Design review of the part built by this model. Coordinates are the model's own, in mm. A direction names the side the tool comes from. Coordinates: 2 decimals unless noted, no trailing zeros. Loops run counter-clockwise (first coordinate to the right, second up) from the corner with the lowest first, then second, coordinate; pieces in that order, holes last. Notation, with made-up numbers: (19, 64) -> (75, 64) arc R4 ccw to (75, 69) -> close; hole circle Ø7 at (81, -4). An arc over 180 degrees is marked (long way). Use one line per item in the form item = value. Start each with the question number.
1. Machinability: for faces 1 (the face through (-6, -0.3, 3)), 2 (the face through (6, 2.2, 3)), 3 (the face through (-6.5, -2.2, 3)), which of the approach directions +Z, -Z, +X, -X, +Y, -Y give a long, thin tool a straight path to every point of the face, cutting with its end or side? Answer none if there is none.
2. Consider section B-B (y = 1). State the section outline as (x, z) points, then the cut area to 3 significant figures.
3. Wall thickness on line 1 (Y direction, x = -9.5, z = 1.25); line 2 (X direction, y = -1.75, z = 4.25); line 3 (Y direction, x = 0.25, z = 3): over which ranges is each line inside the solid? List them lowest first. Write a range as from..to.
4. Consider section A-A (x = 0). State the section outline as (y, z) points, then the cut area to 3 significant figures.
5. The part is to be moulded in two halves that separate along X. For faces 4 (the face through (3, 3, 0)), 5 (the face through (-7.384, -1.237, 1.735)), 6 (the face through (0, 5, 3)), say which applies: released by +X, released by -X, zero draft, split by the parting line, or undercut.
6. Consider section C-C (y = -3). State the section outline as (x, z) points.
7. Consider section D-D (x = -7.5). State the section outline as (y, z) points.
8. For pin 1 (1.8 mm diameter, centred on x = -7, z = 2, fed in from +Y); pin 2 (2.5 mm diameter, centred on x = 8.19, z = 3, fed in from -Y); pin 3 (3.5 mm diameter, centred on x = -8.19, z = 3, fed in from -Y); pin 4 (1.5 mm diameter, centred on y = 1.5, z = 2, fed in from -X), all flat-tipped, find the tip position at first contact; note any pin that passes through.
from build123d import *

# Parameters (mm, degrees)
EXTRUDE_1_DEPTH     = 6
CUT_EXTRUDE_1_DEPTH = 8.2
SKETCH_4_R          = 1.5
CUT_EXTRUDE_2_DEPTH = 8.2
FILLET_1_R          = 0.3


with BuildPart() as part:
    # 草图2 → 凸台-拉伸1 (new body)
    with BuildSketch(Plane.XY):
        with BuildLine():
            Line((-11.189988864, 0.3), (-11.189988864, 2.2))
            Line((-11.189988864, 2.2), (-4.489988864, 2.2))
            ThreePointArc((-4.489988864, 2.2), (0, 5), (4.489988864, 2.2))
            Line((4.489988864, 2.2), (11.189988864, 2.2))
            Line((11.189988864, 2.2), (11.189988864, 0))
            Line((11.189988864, 0), (4, 0))
            ThreePointArc((4, 0), (0.150105729, 3.997182541), (-3.988734135, 0.3))
            Line((-3.988734135, 0.3), (-11.189988864, 0.3))
        make_face()
    extrude_1 = extrude(amount=EXTRUDE_1_DEPTH)

    # 镜向2: 凸台-拉伸1 across plane
    add(extrude_1.mirror(Plane.ZX))

    # 草图3 → 切除-拉伸1 (cut, through all)
    with BuildSketch(Plane(origin=(0, 2.2, 0), x_dir=(1, 0, 0), z_dir=(0, 1, 0))):
        with BuildLine():
            ThreePointArc((-11.189988864, -3), (-10.311309208, -0.878679656), (-8.189988864, 0))
            Line((-8.189988864, 0), (-11.189988864, 0))
            Line((-11.189988864, 0), (-11.189988864, -3))
        make_face()
        with BuildLine():
            ThreePointArc((-8.189988864, -6), (-10.311309208, -5.121320344), (-11.189988864, -3))
            Line((-11.189988864, -3), (-11.189988864, -6))
            Line((-11.189988864, -6), (-8.189988864, -6))
        make_face()
    cut_extrude_1 = extrude(amount=-CUT_EXTRUDE_1_DEPTH, mode=Mode.SUBTRACT)

    # 镜向1: 切除-拉伸1 across plane
    add(cut_extrude_1.mirror(Plane(origin=(0, 0, 0), x_dir=(0, 0, 1), z_dir=(1, 0, 0))), mode=Mode.SUBTRACT)

    # 草图4 → 切除-拉伸2 (cut, through all)
    with BuildSketch(Plane(origin=(0, 2.2, 0), x_dir=(1, 0, 0), z_dir=(0, 1, 0))):
        with Locations((-8.189988864, -3)):
            Circle(SKETCH_4_R)
        with Locations((8.189988864, -3)):
            Circle(SKETCH_4_R)
    extrude(amount=-CUT_EXTRUDE_2_DEPTH, mode=Mode.SUBTRACT)

    # 圆角1
    fillet_1_edges = [part.edges().sort_by_distance(p)[0] for p in [
        (-4.489988864, 2.2, 3),
        (4.489988864, 2.2, 3),
        (-4.489988864, -2.2, 3),
        (4.489988864, -2.2, 3),
    ]]
    fillet(fillet_1_edges, radius=FILLET_1_R)


solid = part.part
Geometry check:
q1.face_1 = +Z, -Z, -X
q1.face_2 = +Z, -Z, +X, +Y
q1.face_3 = +Z, -Z, -X, -Y
q2.outline = (-8.19, 0) -> (-3.87, 0) -> (-3.87, 6) -> (-8.19, 6) arc R3 ccw to start; (3.87, 0) -> (8.19, 0) arc R3 ccw to (8.19, 6) -> (3.87, 6) -> close; hole circle Ø3 at (-8.19, 3); hole circle Ø3 at (8.19, 3)
q2.area = 65.9 mm²
q3.line_1 = -2.2..-0.3, 0.3..2.2
q3.line_2 = -10.92..-9.02, -7.36..-3.6, 3.6..7.36, 9.02..10.92
q3.line_3 = -4.99..-3.99, 3.99..4.99
q4.outline = (-5, 0) -> (-4, 0) -> (-4, 6) -> (-5, 6) -> close; (4, 0) -> (5, 0) -> (5, 6) -> (4, 6) -> close
q4.area = 12.0 mm²
q5.face_4 = zero draft
q5.face_5 = undercut
q5.face_6 = split by the parting line
q6.outline = (-4, 0) -> (-2.65, 0) -> (-2.65, 6) -> (-4, 6) -> close; (2.65, 0) -> (4, 0) -> (4, 6) -> (2.65, 6) -> close
q7.outline = (-2.2, 0) -> (-0.3, 0) -> (-0.3, 1.67) -> (-2.2, 1.67) -> close; (-2.2, 4.33) -> (-0.3, 4.33) -> (-0.3, 6) -> (-2.2, 6) -> close; (0.3, 0) -> (2.2, 0) -> (2.2, 1.67) -> (0.3, 1.67) -> close; (0.3, 4.33) -> (2.2, 4.33) -> (2.2, 6) -> (0.3, 6) -> close
q8.pin_1 = 2.2
q8.pin_2 = through
q8.pin_3 = -2.2
q8.pin_4 = -11.18
